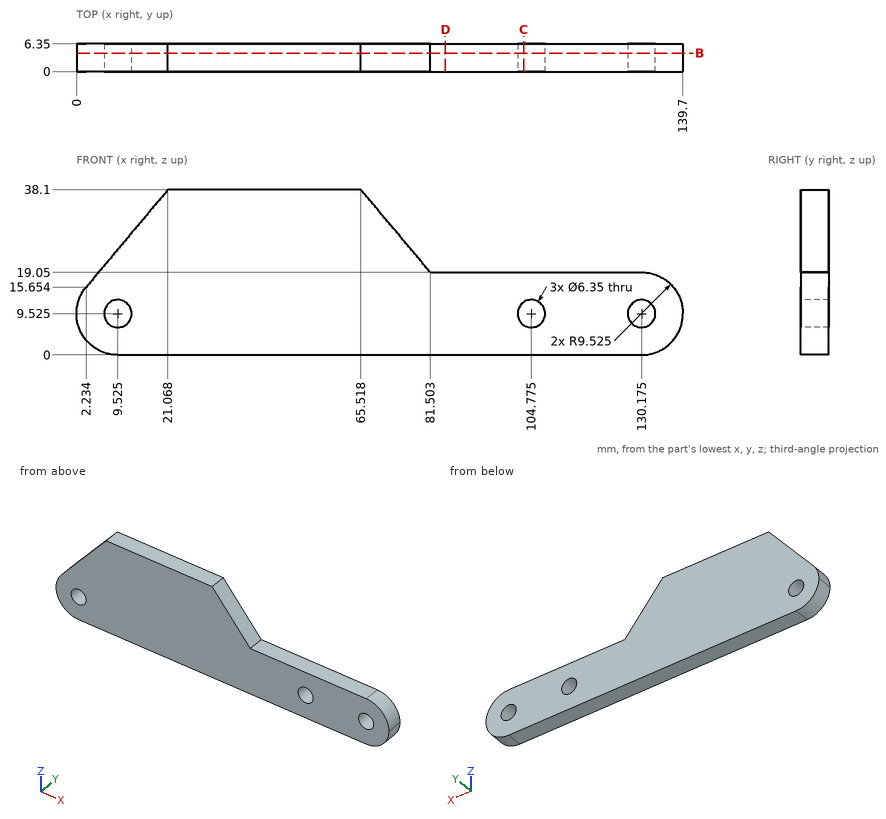
Here's the drawing with two shaded views (mm, measured from the low corner). I have some questions. Coordinates: 2 decimals unless noted, no trailing zeros. Write each loop counter-clockwise with the first axis right and the second up, starting at its lowest first coordinate (ties: lowest second). Pieces come first, ordered by that corner, then holes. Notation, with made-up numbers: (63.25, 21.5) -> (85.25, 21.5) arc R24 cw to (85.25, 45.5) -> close; hole circle Ø1 at (43.5, 68). An arc over 180 degrees is marked (long way). Write item = value, one per line. Start each with the question number.
(1) I need wall thicknesses on line 1 (X direction, y = 1, z = 10) (1 decimal); line 2 (X direction, y = 4, z = 11) (1 decimal); line 3 (Z direction, x = 109.5, y = 3.75). Which ranges of each line are inside material? Lowest first, please. Write a range as [from, to].
(2) Will these pins go through, and if not, where does the flat tip stop? pin 1 (8.5 mm diameter, centred on x = 104.775, z = 9.525, fed in from +Y); pin 2 (1.9 mm diameter, centred on x = 105, y = 2, fed in from +Z); pin 3 (2 mm diameter, centred on y = 5.5, z = 26, fed in from -X) (1 decimal).
(3) I want a section at C-C (x = 103). Please give me the cut outline in (y, z).
(4) I want a section at D-D (x = 85). Please give me the cut outline in (y, z).
(5) I want a section at B-B (y = 4.25). Give the number of separate pieces and of enclosed holes in the cut face, plus the area to 3 significant figures.
Result set:
q1.line_1 = [0, 6.4], [12.7, 101.6], [107.9, 127], [133.3, 139.7]
q1.line_2 = [0.1, 6.7], [12.3, 102], [107.6, 127.4], [133, 139.6]
q1.line_3 = [0, 19.05]
q2.pin_1 = 6.35
q2.pin_2 = 19.05
q2.pin_3 = 10.1
q3.outline = (0, 0) -> (6.35, 0) -> (6.35, 6.89) -> (0, 6.89) -> close; (0, 12.16) -> (6.35, 12.16) -> (6.35, 19.05) -> (0, 19.05) -> close
q4.outline = (0, 0) -> (6.35, 0) -> (6.35, 19.05) -> (0, 19.05) -> close
q5.separate_pieces = 1
q5.enclosed_holes = 3
q5.area = 3,640 mm2
